from build123d import *

# Parameters (mm, degrees)
SKETCH_1_W               = 32
SKETCH_1_H               = 32
EXTRUDE_1_DEPTH          = 1.65
SKETCH_2_W               = 15.425
SKETCH_2_H               = 1.65
SKETCH_3_R               = 12.85
EXTRUDE_2_DEPTH          = 11.25
EXTRUDE_3_DEPTH          = 6.75
PATTERN_CIRCULAR_1_COUNT = 6
FILLET_1_R               = 1
FILLET_2_R               = 1
SKETCH_4_R               = 1.15
CUT_EXTRUDE_2_DEPTH      = 13.9
CHAMFER_1_SIZE           = 0.5


with BuildPart() as part:
    # Sketch 1 → Extrude 1 (new body)
    with BuildSketch(Plane(origin=(0, 0, 0), x_dir=(1, 0, 0), z_dir=(0, 1, 0))):
        Rectangle(SKETCH_1_W, SKETCH_1_H)
    extrude(amount=-EXTRUDE_1_DEPTH)

    # Sketch 2 → Revolve 2 (revolve)
    with BuildSketch(Plane(origin=(0, 0, 0), x_dir=(0, 0, -1), z_dir=(1, 0, 0))):
        with Locations((-7.7125, -0.825)):
            Rectangle(SKETCH_2_W, SKETCH_2_H)
        with BuildLine():
            Line((-15.425, 0), (0, 0))
            ThreePointArc((0, 0), (-5.190857347, 0.326284094), (-10.3, 1.3))
            Line((-10.3, 1.3), (-10.75, 1.3))
            ThreePointArc((-10.75, 1.3), (-11.333421954, 1.670447361), (-12.012265484, 1.8))
            ThreePointArc((-12.012265484, 1.8), (-13.263991109, 1.309826653), (-13.85, 0.1))
            Line((-13.85, 0.1), (-15.425, 0.1))
            Line((-15.425, 0.1), (-15.425, 0))
        make_face()
    revolve(axis=Axis((0, 0, 0), (0, -1, 0)))

    # Sketch 3 → Extrude 2 (add)
    with BuildSketch(Plane.XZ.offset(1.65)):
        Circle(SKETCH_3_R)
    extrude(amount=EXTRUDE_2_DEPTH)

    # Sketch 3_3 → Extrude 3 (add)
    with BuildSketch(Plane.XZ.offset(1.65)):
        with BuildLine():
            ThreePointArc((-3.425, -13.961017155), (0, -14.375), (3.425, -13.961017155))
            Line((3.425, -13.961017155), (3.425, -12.385147355))
            ThreePointArc((3.425, -12.385147355), (0, -12.85), (-3.425, -12.385147355))
            Line((-3.425, -12.385147355), (-3.425, -13.961017155))
        make_face()
        with BuildLine():
            ThreePointArc((-3.425, 12.385147355), (0, 12.85), (3.425, 12.385147355))
            Line((3.425, 12.385147355), (3.425, 13.961017155))
            ThreePointArc((3.425, 13.961017155), (0, 14.375), (-3.425, 13.961017155))
            Line((-3.425, 13.961017155), (-3.425, 12.385147355))
        make_face()
    extrude_3 = extrude(amount=EXTRUDE_3_DEPTH)

    # Pattern Circular 1: Extrude 3 ×6 about axis
    pattern_circular_1_axis = Axis((0, 0, 0), (0, 1, 0))
    for i in range(1, PATTERN_CIRCULAR_1_COUNT):
        add(extrude_3.rotate(pattern_circular_1_axis, i * 360 / PATTERN_CIRCULAR_1_COUNT))

    # Fillet 1
    fillet_1_edges = [part.edges().sort_by_distance(p)[0] for p in [
        (-16, -0.825, 16),
        (-16, -0.825, -16),
        (16, -0.825, -16),
        (16, -0.825, 16),
    ]]
    fillet(fillet_1_edges, radius=FILLET_1_R)

    # Fillet 2
    fillet_2_edges = [part.edges().sort_by_distance(p)[0] for p in [
        (-12.85, -12.9, 0),
    ]]
    fillet(fillet_2_edges, radius=FILLET_2_R)

    # Sketch 4 → Cut-Extrude 2 (cut, through all)
    with BuildSketch(Plane(origin=(0, 0, 0), x_dir=(1, 0, 0), z_dir=(0, 1, 0))):
        with Locations((-12.25, 12.25)):
            Circle(SKETCH_4_R)
        with Locations((12.25, 12.25)):
            Circle(SKETCH_4_R)
        with Locations((12.25, -12.25)):
            Circle(SKETCH_4_R)
        with Locations((-12.25, -12.25)):
            Circle(SKETCH_4_R)
    extrude(amount=-CUT_EXTRUDE_2_DEPTH, mode=Mode.SUBTRACT)

    # Chamfer 1
    chamfer_1_edges = [part.edges().sort_by_distance(p)[0] for p in [
        (0, -8.4, 14.375),
        (0, -8.4, -14.375),
        (-12.449115179, -8.4, 7.1875),
        (12.449115179, -8.4, -7.1875),
        (-12.449115179, -8.4, -7.1875),
        (12.449115179, -8.4, 7.1875),
    ]]
    chamfer(chamfer_1_edges, length=CHAMFER_1_SIZE)


solid = part.part
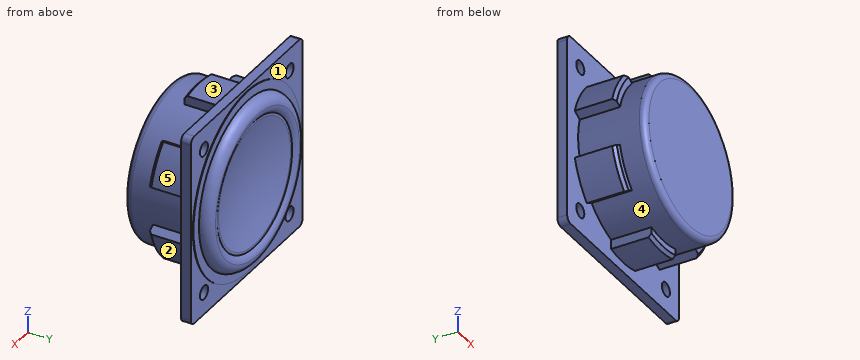
The model under review builds one solid part; all positions refer to its coordinate system, in mm. Face numbers are marked on the shaded views. A direction names the side the tool comes from. Give positions to 0.01 mm unless a question says otherwise; leave off trailing zeros. Order: outer loops, then holes, each group sorted by start corner. A loop starts at its lowest first (then second) coordinate and runs counter-clockwise, first axis right, second up. Notation, with made-up numbers: M 76.25,-26.5 L 121.25,-26.5 A22 cw 121.25,2.5 Z; hole C 0.5,52.5 d9. An arc over 180 degrees is marked long. One line per question, with ' | ' between items. Start each with the question number.
1) Clearance check with flat-ended pins moving along their axes: P1, Ø3, axis at x = 12.25, z = 12.25, coming from the -Y side; P2, Ø9.5, axis at x = 7, z = 2, coming from the +Y side; P3, Ø6, axis at x = -3.5, y = -11, coming from the -Z side; P4, Ø0.7, axis at x = -1, z = -13, coming from the -Y side. State where each tip first meets the part, or that it passes through.
2) Consider section B-B, the plane y = -10.25. Give the boundary of the cut face in (x, z), then the cut area to 3 significant figures.
3) Wall thickness on L1, parallel to X at y = -0.45, z = -12.25; L2, parallel to Y at x = -12, z = -11: over which ranges is each line inside the solid? List them lowest first. Write a range as from..to.
4) Consider section A-A, the plane y = -3.75. Give the boundary of the cut face in (x, z) (3 decimals), then the cut area to 3 significant figures.
5) For the marked faces 1, 2, 3, 4 and 5, list the 3-axis set-ups (+Z, -Z, +X, -X, +Y, -Y) from which the entire face can be reached by the end or side of a thin tool; tool diameter is ignored.
Found:
1) P1: stops at y = -1.65 | P2: stops at y = 1.8 | P3: stops at z = -13.92 | P4: stops at y = -12.45
2) outline: C 0,0 d25.7 | area: 519 mm²
3) L1: x = -16..-13.4, -11.1..11.1, 13.4..16 | L2: y = -1.65..0
4) outline: M -13.803,-4.014 A14.375 ccw -10.378,-9.947 L -9.013,-9.159 A12.85 ccw -3.425,-12.385 L -3.425,-13.961 A14.375 ccw 3.425,-13.961 L 3.425,-12.385 A12.85 ccw 9.013,-9.159 L 10.378,-9.947 A14.375 ccw 13.803,-4.014 L 12.438,-3.226 A12.85 ccw 12.438,3.226 L 13.803,4.014 A14.375 ccw 10.378,9.947 L 9.013,9.159 A12.85 ccw 3.425,12.385 L 3.425,13.961 A14.375 ccw -3.425,13.961 L -3.425,12.385 A12.85 ccw -9.013,9.159 L -10.378,9.947 A14.375 ccw -13.803,4.014 L -12.438,3.226 A12.85 ccw -12.438,-3.226 Z | area: 582 mm²
5) face 1: +Y | face 2: -Z, +X, -Y | face 3: +Z, -Y | face 4: -Y | face 5: +Z, +X, -Y
